Part model, mm, in its own coordinate system. Round coordinates to 2 decimals unless told otherwise and drop trailing zeros. Loops run counter-clockwise (first coordinate to the right, second up) from the corner with the lowest first, then second, coordinate; pieces in that order, holes last. Notation, with made-up numbers: M -40,71.25 L -12,71.25 A15 ccw -12,84.25 Z; hole C 68,69.5 d1. An arc over 180 degrees is marked long. Put each result on its own line as item: value. Start each with the question number.
```python
from build123d import *

# Parameters (mm, degrees)
CYLINDER_R        = 2.25
CYLINDER_DEPTH    = 10
CYLINDER001_R     = 4
CYLINDER001_DEPTH = 25
CYLINDER002_R     = 2.25
CYLINDER002_DEPTH = 10
CYLINDER003_R     = 4
CYLINDER003_DEPTH = 25
PAD_DEPTH         = 15
FILLET_R          = 4


with BuildPart() as cylinder:
    # Cylinder → Cylinder (new body)
    with BuildSketch(Plane.XY):
        Circle(CYLINDER_R)
    extrude(amount=CYLINDER_DEPTH)


with BuildPart() as fusion:
    # Cylinder001 → Cylinder001 (new body)
    with BuildSketch(Plane.XY.offset(2)):
        Circle(CYLINDER001_R)
    extrude(amount=CYLINDER001_DEPTH)

    # Fusion: union Cylinder
    add(cylinder.part)


with BuildPart() as fusion_1:
    # Fusion placement: moved
    add(fusion.part.moved(Location((90, -7.5, 0))))


with BuildPart() as cylinder002:
    # Cylinder002 → Cylinder002 (new body)
    with BuildSketch(Plane.XY):
        Circle(CYLINDER002_R)
    extrude(amount=CYLINDER002_DEPTH)


with BuildPart() as fusion002:
    # Cylinder003 → Cylinder003 (new body)
    with BuildSketch(Plane.XY.offset(2)):
        Circle(CYLINDER003_R)
    extrude(amount=CYLINDER003_DEPTH)

    # Fusion001: union Cylinder002
    add(cylinder002.part)


with BuildPart() as fusion002_1:
    # Fusion001 placement: moved
    add(fusion002.part.moved(Location((-90, -7.5, 0))))

    # Fusion002: union Fusion
    add(fusion_1.part)


with BuildPart() as fillet_body:
    # Sketch → Pad (new body)
    with BuildSketch(Plane.XZ):
        Polygon((-80, 0), (-55, 25), (55, 25), (80, 0), (100, 0), (55, 45), (-55, 45), (-100, 0), align=None)
    extrude(amount=PAD_DEPTH)

    # Cut: cut Fusion002
    add(fusion002_1.part, mode=Mode.SUBTRACT)

    # Fillet
    fillet_edges = [fillet_body.edges().sort_by_distance(p)[0] for p in [
        (-67.5, 0, 12.5),
        (-67.5, -15, 12.5),
        (0, 0, 25),
        (0, -15, 25),
        (67.5, 0, 12.5),
        (77.5, 0, 22.5),
        (0, 0, 45),
        (-77.5, 0, 22.5),
        (67.5, -15, 12.5),
        (77.5, -15, 22.5),
        (0, -15, 45),
        (-77.5, -15, 22.5),
        (-55, -7.5, 45),
        (55, -7.5, 45),
    ]]
    fillet(fillet_edges, radius=FILLET_R)


solid = fillet_body.part
```
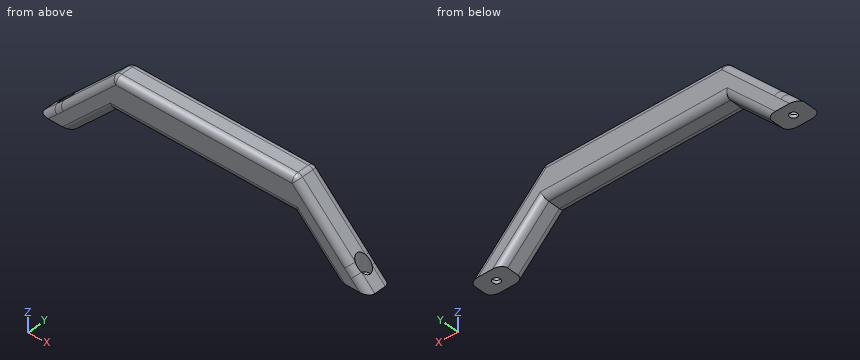
1. Cut at A-A, the plane y = -7.5. Give the cut face in (x, z), and give its area (3 significant figures).
2. Cut at B-B, the plane x = -48.5. Give the cut face in (y, z).
3. Wall check: L1, parallel to Y at x = 90, z = 1; L2, parallel to X at y = -7.5, z = 0.5; L3, parallel to X at y = -7.5, z = 1.55. Give the ranges that are in metal, low to high.
4. Drop flat-ended pins along their axis: pin 1 (5 mm diameter, centred on x = 90, y = -7.5, fed in from +Z); pin 2 (5 mm diameter, centred on x = -10.5, y = -13.5, fed in from +Z); pin 3 (5.5 mm diameter, centred on x = 12, y = -9, fed in from -Z); pin 4 (9 mm diameter, centred on x = -90, y = -9, fed in from +Z). Give the stop position or say it passes through.
Results list:
1. outline: M -100,0 L -92.25,0 L -92.25,2 L -94,2 L -94,6 Z; M -87.75,0 L -80,0 L -55,25 L 55,25 L 80,0 L 87.75,0 L 87.75,2 L 86,2 L 86,14 L 56.17,43.83 A4 ccw 53.34,45 L -53.34,45 A4 ccw -56.17,43.83 L -86,14 L -86,2 L -87.75,2 Z; M 92.25,0 L 100,0 L 94,6 L 94,2 L 92.25,2 Z
1. area: 3,450 mm^2
2. outline: M -15,29 A4 ccw -11,25 L -4,25 A4 ccw 0,29 L 0,41 A4 ccw -4,45 L -11,45 A4 ccw -15,41 Z
3. L1: y = -15 to -9.75, -5.25 to 0
3. L2: x = -99.5 to -92.25, -87.75 to -79.5, 79.5 to 87.75, 92.25 to 99.5
3. L3: x = -98.45 to -92.25, -87.75 to -78.45, 78.45 to 87.75, 92.25 to 98.45
4. pin 1: stops at z = 2
4. pin 2: stops at z = 45
4. pin 3: stops at z = 25
4. pin 4: stops at z = 14.5
